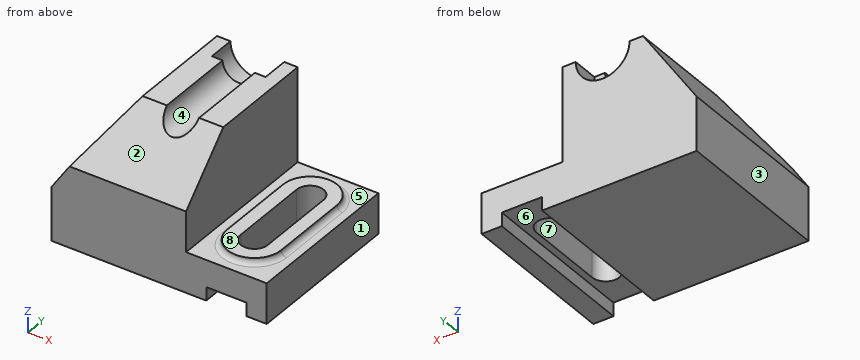
from build123d import *

# Parameters (mm, degrees)
F0_W         = 80
F0_H         = 60
F1_DEPTH     = 50
F2_W         = 30
F2_H         = 33
F3_DEPTH     = 60.001
F5_DEPTH     = 17.001
F6_W         = 30
F6_H         = 60
F7_DEPTH     = 2
F8_W         = 15
F8_H         = 5
F9_DEPTH     = 60.001
F10_R        = 1.99999
F12_DEPTH    = 60.001
F13_W        = 6
F13_H        = 48.9288835973
F15_W        = 4
F15_H        = 10
F17_T1_DEPTH = 132.8673195186


# Not quite as in the source:
# - a fillet or chamfer that OpenCascade refuses, or shapes differently, is made with other operations: its cross-section is extruded or revolved along the edge and cut away or added
# - a fillet or chamfer is up to 0.001 mm smaller than in the source, because OpenCascade refuses the exact size


with BuildPart() as f1:
    # F0 (on Top) → F1 (new body)
    with BuildSketch(Plane.XY):
        Rectangle(F0_W, F0_H)
    extrude(amount=F1_DEPTH)

    # F2 (on face) → F3 (cut, through all)
    with BuildSketch(Plane.XZ.offset(30)):
        with Locations((25, 33.5)):
            Rectangle(F2_W, F2_H)
    extrude(amount=-F3_DEPTH, mode=Mode.SUBTRACT)

    # F4 (on face) → F5 (cut, through all)
    with BuildSketch(Plane.XY.offset(17)):
        with BuildLine():
            ThreePointArc((20, -15), (25, -20), (30, -15))
            Line((30, -15), (30, 15))
            ThreePointArc((30, 15), (25, 20), (20, 15))
            Line((20, 15), (20, -15))
        make_face()
    extrude(amount=-F5_DEPTH, mode=Mode.SUBTRACT)

    # F6 (on face) → F7 (cut)
    with BuildSketch(Plane.XY.offset(17)):
        with Locations((25, 0)):
            Rectangle(F6_W, F6_H)
        with BuildLine():
            Line((35, 15), (35, -15))
            ThreePointArc((35, -15), (25, -25), (15, -15))
            Line((15, -15), (15, 15))
            ThreePointArc((15, 15), (25, 25), (35, 15))
        make_face(mode=Mode.SUBTRACT)
    extrude(amount=-F7_DEPTH, mode=Mode.SUBTRACT)

    # F8 (on face) → F9 (cut, through all)
    with BuildSketch(Plane.XZ.offset(30)):
        with Locations((25, 2.5)):
            Rectangle(F8_W, F8_H)
    extrude(amount=-F9_DEPTH, mode=Mode.SUBTRACT)

    # F10 (radius 2 in the source; OpenCascade refuses exactly that, so slightly less here)
    f10_edges = [f1.edges().sort_by_distance(p)[0] for p in [
        (35, 0, 15),
    ]]
    fillet(f10_edges, radius=F10_R)

    # F11 (on face) → F12 (cut, through all)
    with BuildSketch(Plane.XZ.offset(30)):
        Polygon((-40, 20), (-20, 50), (-40, 50), align=None)
    extrude(amount=-F12_DEPTH, mode=Mode.SUBTRACT)

    # F13 (on face) → F14 (revolve, cut)
    with BuildSketch(Plane.XY.offset(50)):
        with Locations((-8, 5.5355582014)):
            Rectangle(F13_W, F13_H)
    revolve(axis=Axis((-5, -1.603256911, 50), (0, -1, 0)), mode=Mode.SUBTRACT)

    # F15 (on face) → F16 (revolve, cut)
    with BuildSketch(Plane.XY.offset(50)):
        with Locations((-13, 25)):
            Rectangle(F15_W, F15_H)
    revolve(axis=Axis((-5, 25, 50), (0, -1, 0)), mode=Mode.SUBTRACT)

    # F17: chamfer of 20 on 1 edges, made by hand

    # F17_s2 → F17_t1 (cut)
    with BuildSketch(Plane.YZ.offset(-71.4336597593)):
        Polygon((-30, 30), (-10, 50), (-30, 50), align=None)
    extrude(amount=F17_T1_DEPTH, mode=Mode.SUBTRACT)


solid = f1.part
The model under review builds one solid part; all positions refer to its coordinate system, in mm. Face numbers are marked on the shaded views. A direction names the side the tool comes from. Give positions to 0.01 mm unless a question says otherwise; leave off trailing zeros. Loops run counter-clockwise (first coordinate to the right, second up) from the corner with the lowest first, then second, coordinate; pieces in that order, holes last. Notation, with made-up numbers: (78.5, 30.5) -> (82.5, 30.5) arc R33 ccw to (82.5, 69.5) -> close; hole circle Ø5 at (37, -30.75). An arc over 180 degrees is marked (long way). Put each result on its own line as item: value. Start each with the question number.
1. Clearance check with flat-ended pins moving along their axes: P1, Ø1.5, axis at x = -9, y = 1.5, coming from the +Z side; P2, Ø24, axis at x = 24.5, y = 5.5, coming from the +Z side; P3, Ø2, axis at y = 16.5, z = 42.5, coming from the -X side. State where each tip first meets the part, or that it passes through.
2. We need section B-B on z = 16. State the section outline as (x, y) points.
3. We need section D-D on x = -5. State the section outline as (y, z) points.
4. Mouldability with a two-part tool opening along X and no side actions: class the marked faces 1, 2, 3 and 4 as released by +X, released by -X, zero draft, split by the parting line, or undercut.
5. Wall thickness on probe 1 along Z at (x, y) = (28, -24); probe 2 along X at (y, z) = (-1.5, 42.5); probe 3 along Z at (x, y) = (-4.5, 7): over which ranges is each line inside the solid? List them lowest first.
6. For the marked faces 5, 6, 7 and 8, list the 3-axis set-ups (+Z, -Z, +X, -X, +Y, -Y) from which the entire face can be reached by the end or side of a thin tool; tool diameter is ignored.
Determined:
1. P1: z = 46.33
1. P2: z = 17
1. P3: x = -25.67
2. outline: (-40, -30) -> (10, -30) -> (10, 30) -> (-40, 30) -> close; (14.73, -15) arc R10.27 ccw to (35.27, -15) -> (35.27, 15) arc R10.27 ccw to (14.73, 15) -> close; hole (20, -15) arc R5 ccw to (30, -15) -> (30, 15) arc R5 ccw to (20, 15) -> close
3. outline: (-30, 0) -> (30, 0) -> (30, 40) -> (20, 40) -> (20, 44) -> (-16, 44) -> (-30, 30) -> close
4. face 1: released by +X
4. face 2: zero draft
4. face 3: released by -X
4. face 4: undercut
5. probe 1: 5 to 17
5. probe 2: -25 to 10
5. probe 3: 0 to 44.02
6. face 5: +Z
6. face 6: -Z, +Y, -Y
6. face 7: +Z, -Z
6. face 8: +Z, +X, +Y, -Y
